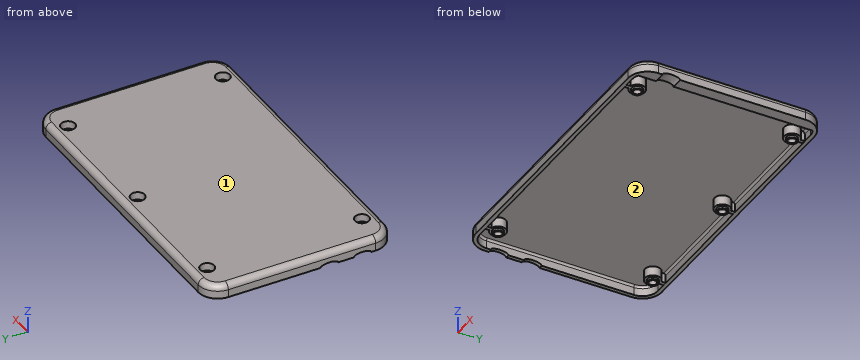
```python
from build123d import *

# Parameters (mm, degrees)
BOSS_EXTRUDE1_DEPTH                             = 8.89
FILLET1_R                                       = 3.81
SHELL1_T                                        = -2.54
BOSS_EXTRUDE4_REACH                             = 10.89
BOSS_EXTRUDE2_REACH                             = 10.763
SKETCH3_R                                       = 3.5052
BOSS_EXTRUDE3_DEPTH                             = 1.5875
CBORE_FOR_8_PAN_HEAD_MACHINE_SCREW1_D           = 4.9149
CBORE_FOR_8_PAN_HEAD_MACHINE_SCREW1_CBORE_D     = 9.12876
CBORE_FOR_8_PAN_HEAD_MACHINE_SCREW1_CBORE_DEPTH = 5.08
CUT_EXTRUDE1_REACH                              = 205.12
CUT_EXTRUDE3_REACH                              = 205.12
CUT_EXTRUDE4_REACH                              = 205.12


with BuildPart() as part:
    # Sketch1 → Boss-Extrude1 (new body)
    with BuildSketch(Plane.XY):
        with BuildLine():
            Line((5.08, 103.26), (5.08, 21.725))
            Line((5.08, 21.725), (5.08, 7.5))
            ThreePointArc((5.08, 7.5), (1.395403307, -1.395403307), (-7.5, -5.08))
            Line((-7.5, -5.08), (-185.46, -5.08))
            ThreePointArc((-185.46, -5.08), (-194.355403307, -1.395403307), (-198.04, 7.5))
            Line((-198.04, 7.5), (-198.04, 103.26))
            ThreePointArc((-198.04, 103.26), (-194.355403307, 112.155403307), (-185.46, 115.84))
            Line((-185.46, 115.84), (-7.5, 115.84))
            ThreePointArc((-7.5, 115.84), (1.395403307, 112.155403307), (5.08, 103.26))
        make_face()
    extrude(amount=BOSS_EXTRUDE1_DEPTH)

    # Fillet1
    fillet1_edges = [part.edges().sort_by_distance(p)[0] for p in [
        (-96.48, -5.08, 8.89),
        (1.395403307, -1.395403307, 8.89),
        (5.08, 55.38, 8.89),
        (1.395403307, 112.155403307, 8.89),
        (-96.48, 115.84, 8.89),
        (-194.355403307, 112.155403307, 8.89),
        (-198.04, 55.38, 8.89),
        (-194.355403307, -1.395403307, 8.89),
    ]]
    fillet(fillet1_edges, radius=FILLET1_R)

    # Shell1
    shell1_openings = [part.faces().sort_by_distance(p)[0] for p in [
        (-96.48, 55.38, 0),
    ]]
    offset(amount=SHELL1_T, openings=shell1_openings, kind=Kind.INTERSECTION)

    # Sketch7 → Boss-Extrude4 (add, up to next)
    with BuildSketch(Plane(origin=(0, 0, 0), x_dir=(-1, 0, 0), z_dir=(0, 0, -1)), mode=Mode.PRIVATE) as boss_extrude4_sk1:
        with BuildLine():
            Line((-2.54, 7.5), (-2.54, 103.26))
            ThreePointArc((-2.54, 103.26), (-1.17755726, 108.30991089), (2.54, 111.989261137))
            Line((2.54, 111.989261137), (2.54, 95.52))
            Line((2.54, 95.52), (2.54, 92.98))
            Line((2.54, 92.98), (2.54, 21.725))
            Line((2.54, 21.725), (2.54, 10.295))
            Line((2.54, 10.295), (2.54, -1.229261137))
            ThreePointArc((2.54, -1.229261137), (-1.17755726, 2.45008911), (-2.54, 7.5))
        make_face()
    boss_extrude4_tool1 = extrude(boss_extrude4_sk1.sketch, amount=-BOSS_EXTRUDE4_REACH, mode=Mode.PRIVATE) - part.part
    add(boss_extrude4_tool1.solids().sort_by_distance((-0.052284, 55.38, 0))[0])

    # Sketch2 → Boss-Extrude2 (add, up to next)
    with BuildSketch(Plane(origin=(0, 0, 0.127), x_dir=(-1, 0, 0), z_dir=(0, 0, -1)), mode=Mode.PRIVATE) as boss_extrude2_sk1:
        with BuildLine():
            Line((13.97, 110.59868885), (13.97, 113.3))
            Line((13.97, 113.3), (16.51, 113.3))
            Line((16.51, 113.3), (16.51, 110.59868885))
            ThreePointArc((16.51, 110.59868885), (15.24, 100.6), (13.97, 110.59868885))
        make_face()
    boss_extrude2_tool1 = extrude(boss_extrude2_sk1.sketch, amount=-BOSS_EXTRUDE2_REACH, mode=Mode.PRIVATE) - part.part
    add(boss_extrude2_tool1.solids().sort_by_distance((-15.24, 106.155134, 0.127))[0])
    # Sketch2 → Boss-Extrude2 (add, up to next)
    with BuildSketch(Plane(origin=(0, 0, 0.127), x_dir=(-1, 0, 0), z_dir=(0, 0, -1)), mode=Mode.PRIVATE) as boss_extrude2_sk2:
        with BuildLine():
            Line((95.21, 110.59868885), (95.21, 113.3))
            Line((95.21, 113.3), (97.75, 113.3))
            Line((97.75, 113.3), (97.75, 110.59868885))
            ThreePointArc((97.75, 110.59868885), (96.48, 100.6), (95.21, 110.59868885))
        make_face()
    boss_extrude2_tool2 = extrude(boss_extrude2_sk2.sketch, amount=-BOSS_EXTRUDE2_REACH, mode=Mode.PRIVATE) - part.part
    add(boss_extrude2_tool2.solids().sort_by_distance((-96.48, 106.155134, 0.127))[0])
    # Sketch2 → Boss-Extrude2 (add, up to next)
    with BuildSketch(Plane(origin=(0, 0, 0.127), x_dir=(-1, 0, 0), z_dir=(0, 0, -1)), mode=Mode.PRIVATE) as boss_extrude2_sk3:
        with BuildLine():
            Line((176.45, 110.59868885), (176.45, 113.3))
            Line((176.45, 113.3), (178.99, 113.3))
            Line((178.99, 113.3), (178.99, 110.59868885))
            ThreePointArc((178.99, 110.59868885), (177.72, 100.6), (176.45, 110.59868885))
        make_face()
    boss_extrude2_tool3 = extrude(boss_extrude2_sk3.sketch, amount=-BOSS_EXTRUDE2_REACH, mode=Mode.PRIVATE) - part.part
    add(boss_extrude2_tool3.solids().sort_by_distance((-177.72, 106.155134, 0.127))[0])
    # Sketch2 → Boss-Extrude2 (add, up to next)
    with BuildSketch(Plane(origin=(0, 0, 0.127), x_dir=(-1, 0, 0), z_dir=(0, 0, -1)), mode=Mode.PRIVATE) as boss_extrude2_sk4:
        with BuildLine():
            Line((176.45, -2.54), (176.45, 0.16131115))
            ThreePointArc((176.45, 0.16131115), (177.72, 10.16), (178.99, 0.16131115))
            Line((178.99, 0.16131115), (178.99, -2.54))
            Line((178.99, -2.54), (176.45, -2.54))
        make_face()
    boss_extrude2_tool4 = extrude(boss_extrude2_sk4.sketch, amount=-BOSS_EXTRUDE2_REACH, mode=Mode.PRIVATE) - part.part
    add(boss_extrude2_tool4.solids().sort_by_distance((-177.72, 4.604866, 0.127))[0])
    # Sketch2 → Boss-Extrude2 (add, up to next)
    with BuildSketch(Plane(origin=(0, 0, 0.127), x_dir=(-1, 0, 0), z_dir=(0, 0, -1)), mode=Mode.PRIVATE) as boss_extrude2_sk5:
        with BuildLine():
            Line((13.97, -2.54), (13.97, 0.16131115))
            ThreePointArc((13.97, 0.16131115), (15.24, 10.16), (16.51, 0.16131115))
            Line((16.51, 0.16131115), (16.51, -2.54))
            Line((16.51, -2.54), (13.97, -2.54))
        make_face()
    boss_extrude2_tool5 = extrude(boss_extrude2_sk5.sketch, amount=-BOSS_EXTRUDE2_REACH, mode=Mode.PRIVATE) - part.part
    add(boss_extrude2_tool5.solids().sort_by_distance((-15.24, 4.604866, 0.127))[0])

    # Sketch3 → Boss-Extrude3 (add)
    with BuildSketch(Plane(origin=(0, 0, 0.127), x_dir=(-1, 0, 0), z_dir=(0, 0, -1))):
        with Locations((15.24, 105.68)):
            Circle(SKETCH3_R)
        with Locations((96.48, 105.68)):
            Circle(SKETCH3_R)
        with Locations((177.72, 105.68)):
            Circle(SKETCH3_R)
        with Locations((177.72, 5.08)):
            Circle(SKETCH3_R)
        with Locations((15.24, 5.08)):
            Circle(SKETCH3_R)
    extrude(amount=BOSS_EXTRUDE3_DEPTH)

    # CBORE for #8 Pan Head Machine Screw1 (through all)
    with Locations(Plane(origin=(-15.24, 5.08, 8.89), x_dir=(0, 1, 0), z_dir=(0, 0, 1))):
        with Locations((0, 0), (0, 162.48), (100.6, 162.48), (100.6, 81.24), (100.6, 0)):
            CounterBoreHole(CBORE_FOR_8_PAN_HEAD_MACHINE_SCREW1_D / 2, CBORE_FOR_8_PAN_HEAD_MACHINE_SCREW1_CBORE_D / 2, CBORE_FOR_8_PAN_HEAD_MACHINE_SCREW1_CBORE_DEPTH)

    # Sketch5 → Cut-Extrude1 (cut, up to next)
    with BuildSketch(Plane(origin=(-198.04, 192.96, 0), x_dir=(0, 1, 0), z_dir=(1, 0, 0)), mode=Mode.PRIVATE) as cut_extrude1_sk1:
        with BuildLine():
            Line((-171.235, 0), (-182.665, 0))
            add(Edge.make_bspline(
                [(-171.235, 0), (-171.235, 1.905), (-176.95, 1.905), (-182.665, 1.905), (-182.665, 0)],
                knots=[3.141592654, 3.141592654, 3.141592654, 4.71238898, 4.71238898, 6.283185307, 6.283185307, 6.283185307], degree=2, weights=[1, 0.707106781, 1, 0.707106781, 1]))
        make_face()
    cut_extrude1_tool1 = extrude(cut_extrude1_sk1.sketch, amount=CUT_EXTRUDE1_REACH, mode=Mode.PRIVATE) & part.part
    add(cut_extrude1_tool1.solids().sort_by_distance((-198.04, 16.01, 0.808344))[0], mode=Mode.SUBTRACT)

    # Sketch6 → Cut-Extrude3 (cut, up to next)
    with BuildSketch(Plane(origin=(5.08, -160.94, 0), x_dir=(0, -1, 0), z_dir=(-1, 0, 0)), mode=Mode.PRIVATE) as cut_extrude3_sk1:
        with BuildLine():
            Line((-171.235, 0), (-182.665, 0))
            add(Edge.make_bspline(
                [(-171.235, 0), (-171.235, 1.905), (-176.95, 1.905), (-182.665, 1.905), (-182.665, 0)],
                knots=[3.141592654, 3.141592654, 3.141592654, 4.71238898, 4.71238898, 6.283185307, 6.283185307, 6.283185307], degree=2, weights=[1, 0.707106781, 1, 0.707106781, 1]))
        make_face()
    cut_extrude3_tool1 = extrude(cut_extrude3_sk1.sketch, amount=CUT_EXTRUDE3_REACH, mode=Mode.PRIVATE) & part.part
    add(cut_extrude3_tool1.solids().sort_by_distance((5.08, 16.01, 0.808344))[0], mode=Mode.SUBTRACT)

    # Sketch8 → Cut-Extrude4 (cut, up to next)
    with BuildSketch(Plane(origin=(-198.04, -139.35, 0), x_dir=(0, -1, 0), z_dir=(-1, 0, 0)), mode=Mode.PRIVATE) as cut_extrude4_sk1:
        with BuildLine():
            Line((-171.235, 0), (-182.665, 0))
            add(Edge.make_bspline(
                [(-171.235, 0), (-171.235, 1.905), (-176.95, 1.905), (-182.665, 1.905), (-182.665, 0)],
                knots=[3.141592654, 3.141592654, 3.141592654, 4.71238898, 4.71238898, 6.283185307, 6.283185307, 6.283185307], degree=2, weights=[1, 0.707106781, 1, 0.707106781, 1]))
        make_face()
    cut_extrude4_tool1 = extrude(cut_extrude4_sk1.sketch, amount=-CUT_EXTRUDE4_REACH, mode=Mode.PRIVATE) & part.part
    add(cut_extrude4_tool1.solids().sort_by_distance((-198.04, 37.6, 0.808344))[0], mode=Mode.SUBTRACT)


solid = part.part
```
Check sheet for the modelled part. Datum: model origin and axes. Units: mm. Face numbers are marked on the shaded views. Give positions to 0.01 mm unless a question says otherwise; leave off trailing zeros. Write each loop counter-clockwise with the first axis right and the second up, starting at its lowest first coordinate (ties: lowest second). Pieces come first, ordered by that corner, then holes.
Item 1: Cross-section at A-A (y = 71.5). Enter the section's corners in (x, z), and give its area (3 significant figures).
Item 2: Cross-section at B-B (x = -66). Enter the section's corners in (y, z).
Item 3: Scan lines: L1, parallel to Y at x = -177.72, z = 2; L2, parallel to X at y = 37, z = 3.25; L3, parallel to Y at x = -121, z = 2.5. Record each from-to range of solid material in increasing order.
Item 4: Cross-section at C-C (y = 105.68). Count the separate pieces of the cut face and the enclosed holes in it, and give its area (3 significant figures).
Item 5: Gauge pin test, flat ends, axial feed: pin 1 (1.4 mm diameter, centred on y = 111.5, z = 2.5, fed in from +X); pin 2 (1.5 mm diameter, centred on y = 63, z = 7.5, fed in from +X); pin 3 (0.8 mm diameter, centred on y = 112, z = 2, fed in from -X). Record the tip position at first contact, or that the pin passes through.
Item 6: Draft check along Y on the marked faces 1 and 2. Enter one of: released by +Y, released by -Y, zero draft, split by the parting line, or undercut.
Report:
1. outline: (-198.04, 0) - (-195.5, 0) - (-195.5, 5.08) arc R1.27 cw to (-194.23, 6.35) - (-2.54, 6.35) - (-2.54, 0) - (5.08, 0) - (5.08, 5.08) arc R3.81 ccw to (1.27, 8.89) - (-194.23, 8.89) arc R3.81 ccw to (-198.04, 5.08) - close
1. area: 575 mm2
2. outline: (-5.08, 0) - (-2.54, 0) - (-2.54, 5.08) arc R1.27 cw to (-1.27, 6.35) - (112.03, 6.35) arc R1.27 cw to (113.3, 5.08) - (113.3, 0) - (115.84, 0) - (115.84, 5.08) arc R3.81 ccw to (112.03, 8.89) - (-1.27, 8.89) arc R3.81 ccw to (-5.08, 5.08) - close
3. L1: y = -5.08 to 2.62, 7.54 to 10.16, 100.6 to 103.22, 108.14 to 115.84
3. L2: x = -198.04 to -195.5, -2.54 to 5.08
3. L3: y = -5.08 to -2.54, 113.3 to 115.84
4. separate pieces: 4
4. enclosed holes: 0
4. area: 578 mm2
5. pin 1: stops at x = 2.57
5. pin 2: stops at x = 4.69
5. pin 3: stops at x = -194.88
6. face 1: zero draft
6. face 2: undercut
